Geometry: final body of the model. Coordinates: model frame, mm. A direction names the side the tool comes from. Coordinates: 2 decimals unless noted, no trailing zeros. Loops run counter-clockwise (first coordinate to the right, second up) from the corner with the lowest first, then second, coordinate; pieces in that order, holes last. Notation, with made-up numbers: (26.5, 39) - (61.5, 39) arc R30 ccw to (61.5, 78) - close; hole circle Ø5 at (-14, 52). An arc over 180 degrees is marked (long way). Put each result on its own line as item: value. Start each with the question number.
1) Section C-C on x = -20.1. Output: boundary loops of the cut face in (y, z).
2) Section D-D on z = 3.25. Output: boundary loops of the cut face in (x, y) (3 decimals).
3) Draft query along Y for faces 5 (the cylindrical face through (0.18, -3.179, 1.805)), 6 (the cylindrical face through (6.918, -0.837, 0.749)), 7 (the flat face through (5, -12, 8.04)). Return one class per face: +Y half, -Y half, draft (parallel to the pull), parting line (faces both ways), or undercut.
4) Material intervals for line 1 along X through (y, z) = (-12.5, 7.75); line 2 along Y through (x, z) = (29.9, 7.35); line 3 along Z through (x, y) = (-8, 2), sorted ascending. Write a range as from..to.
5) Section A-A on x = 4.9. Output: boundary loops of the cut face in (y, z) (3 decimals), and give its area (3 significant figures).
6) Reachability of faces 1 (the flat face through (0, 1, 1.52)), 2 (the flat face through (0, -5, 2)), 3 (the flat face through (-18.9, -11.9, 6.52)), 4 (the flat face through (0, 5, 1)) from +Z, -Z, +X, -X, +Y, -Y: full face, straight path, thin tool, end or side. Return the list, or none.
7) Section B-B on y = 0. Output: boundary loops of the cut face in (x, z) (3 decimals), and give its area (3 significant figures).
8) Contact query for flat-ended pins moving along their axis: pin 1 Ø4 at (x, y) = (23.5, -13.5) entering from -Z; pin 2 Ø3 at (y, z) = (-7, 5) entering from +X (3 decimals); pin 3 Ø4 at (x, y) = (4.5, -11) entering from -Z. Output: stop coordinate, or through.
```python
from build123d import *

# Parameters (mm, degrees)
SKETCH1_W           = 25.77
SKETCH1_H           = 10
SKETCH1_R           = 2.185
BOSS_EXTRUDE1_DEPTH = 1.52
SKETCH2_W           = 25.77
SKETCH2_H           = 1.52
BOSS_EXTRUDE2_DEPTH = 5
SKETCH3_W           = 25.77
SKETCH3_H           = 1.52
BOSS_EXTRUDE3_DEPTH = 10
BOSS_EXTRUDE4_DEPTH = 1.52
SKETCH5_R           = 1.09
CUT_EXTRUDE1_DEPTH  = 5
FILLET1_R           = 1


with BuildPart() as part:
    # Sketch1 → Boss-Extrude1 (new body)
    with BuildSketch(Plane.XY):
        Rectangle(SKETCH1_W, SKETCH1_H)
        with Locations((-4.9, 0)):
            Circle(SKETCH1_R, mode=Mode.SUBTRACT)
        with Locations((4.9, 0)):
            Circle(SKETCH1_R, mode=Mode.SUBTRACT)
    extrude(amount=BOSS_EXTRUDE1_DEPTH)

    # Sketch2 → Boss-Extrude2 (add)
    with BuildSketch(Plane.XY.offset(1.52)):
        with Locations((0, -4.24)):
            Rectangle(SKETCH2_W, SKETCH2_H)
    extrude(amount=BOSS_EXTRUDE2_DEPTH)

    # Sketch3 → Boss-Extrude3 (add)
    with BuildSketch(Plane(origin=(0, -5, 0), x_dir=(-1, 0, 0), z_dir=(0, -1, 0))):
        with Locations((0, -5.76)):
            Rectangle(SKETCH3_W, SKETCH3_H)
    extrude(amount=BOSS_EXTRUDE3_DEPTH)

    # Sketch4 → Boss-Extrude4 (add)
    with BuildSketch(Plane.XY.offset(6.52)):
        Polygon((-12.885, -15), (-25.1, -15), (-25.1, -10), (34.9, -10), (34.9, -15), align=None)
    extrude(amount=BOSS_EXTRUDE4_DEPTH)

    # Sketch5 → Cut-Extrude1 (cut, symmetric)
    with BuildSketch(Plane.XY.offset(6.52)):
        with Locations(Location((-20.1, -12.5, 0), (0, 0, 180))):
            Circle(SKETCH5_R)
        with Locations(Location((29.9, -12.5, 0), (0, 0, 180))):
            Circle(SKETCH5_R)
    extrude(amount=CUT_EXTRUDE1_DEPTH, both=True, mode=Mode.SUBTRACT)

    # Fillet1
    fillet1_edges = [part.edges().sort_by_distance(p)[0] for p in [
        (0, -5, 0),
        (0, -5, 5),
        (-25.1, -15, 7.28),
        (-25.1, -10, 7.28),
        (34.9, -15, 7.28),
        (34.9, -10, 7.28),
        (0, -10, 6.52),
        (0, -3.48, 6.52),
        (0, -3.48, 1.52),
        (-12.885, 5, 0.76),
        (12.885, 5, 0.76),
        (0, -15, 5),
    ]]
    fillet(fillet1_edges, radius=FILLET1_R)


solid = part.part
```
Answer block:
1. outline: (-15, 6.52) - (-13.59, 6.52) - (-13.59, 8.04) - (-15, 8.04) - close; (-11.41, 6.52) - (-10, 6.52) - (-10, 8.04) - (-11.41, 8.04) - close
2. outline: (-12.885, -5) - (12.885, -5) - (12.885, -3.48) - (-12.885, -3.48) - close
3. face 5: +Y half
3. face 6: undercut
3. face 7: draft
4. line 1: x = -25.1..-21.19, -19.01..28.81, 30.99..34.9
4. line 2: y = -15..-13.59, -11.41..-10
4. line 3: z = 0..1.52
5. outline: (-15, 6) arc R1 ccw to (-14, 5) - (-6, 5) arc R1 cw to (-5, 4) - (-5, 1) arc R1 ccw to (-4, 0) - (-2.185, 0) - (-2.185, 1.52) - (-2.48, 1.52) arc R1 cw to (-3.48, 2.52) - (-3.48, 5.52) arc R1 ccw to (-4.48, 6.52) - (-9, 6.52) arc R1 cw to (-10, 7.52) - (-10, 8.04) - (-15, 8.04) - close; (2.185, 0) - (5, 0) - (5, 1.52) - (2.185, 1.52) - close
5. area: 39.0 mm²
6. face 1: +Z, +X, -X, +Y
6. face 2: -Z, +X, -X, -Y
6. face 3: -Z, -X, +Y, -Y
6. face 4: +Z, -Z, +X, -X, +Y
7. outline: (-12.885, 0) - (-7.085, 0) - (-7.085, 1.52) - (-12.885, 1.52) - close; (-2.715, 0) - (2.715, 0) - (2.715, 1.52) - (-2.715, 1.52) - close; (7.085, 0) - (12.885, 0) - (12.885, 1.52) - (7.085, 1.52) - close
7. area: 25.9 mm²
8. pin 1: stops at z = 6.52
8. pin 2: stops at x = 12.885
8. pin 3: stops at z = 5
